Can you work these out from the model? Positions are in its coordinate system, mm. Give positions to 0.01 mm unless a question says otherwise; leave off trailing zeros. Return JSON: item names as keys, results as strings. Group by question number.
Q1. Will this pin go through, and if not, where does the flat tip stop? pin 1 (2 mm diameter, centred on x = 0, y = 85, fed in from +Z).
Q2. I need wall thicknesses on line 1 along X through (y, z) = (335, -0.35); line 2 along X through (y, z) = (59.5, 0.9). Which ranges of each line are inside material? Lowest first, please. Write a range as [from, to].
Q3. Suppose I cut it at A-A, the plane z = 0.4. Count the separate pieces of the cut face and the enclosed holes in it, and give its area (3 significant figures).
Solid Edge part; units mm, degrees
sketch "Sketch1" plane through (0, 0, 0) normal (0, -1, 0) x (1, 0, 0)
  line L0 (-4.5, -1.25) -> (4.5, -1.25)
  line L1 (4.5, -1.25) -> (4.5, 1.25)
  line L2 (4.5, 1.25) -> (-4.5, 1.25)
  line L3 (-4.5, 1.25) -> (-4.5, -1.25)
  dimension "D1" = 4.5
  dimension "D2" = 4.5
extrude "Protrusion1" add sketch "Sketch1" against normal blind 400
hole "Hole_1" at (0, 10, 1.25) direction (0, 0, -1) diameter 2.459 end up to next
pattern_linear "Pattern1" count 16 spacing 25 along (0, 1, 0) of "Hole_1"
properties material "Stainless Steel, 304"
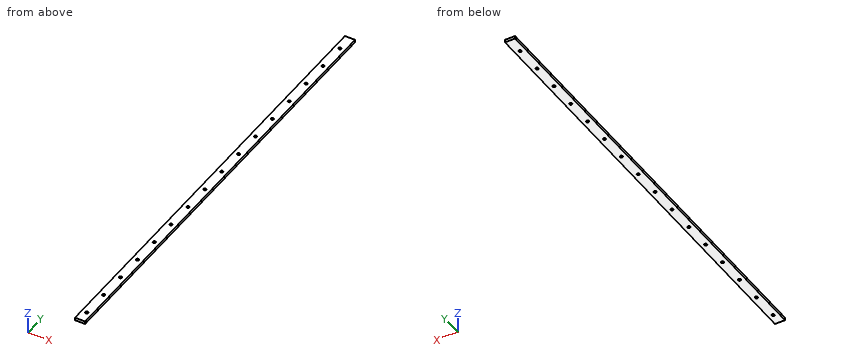
Ans:
{
 "1": {"pin 1": "passes through"},
 "2": {"line 1": "x = [-4.5, -1.23], [1.23, 4.5]", "line 2": "x = [-4.5, -1.12], [1.12, 4.5]"},
 "3": {"separate pieces": "1", "enclosed holes": "16", "area": "3,520 mm^2"}
}
